from build123d import *

# Parameters (mm, degrees)
SKETCH1_R                        = 20
BOSS_EXTRUDE1_DEPTH              = 40
SKETCH1_3_R                      = 20
BOSS_EXTRUDE2_DEPTH              = 30
SKETCH2_W                        = 80
SKETCH2_H                        = 40
BOSS_EXTRUDE3_DEPTH              = 10
SKETCH6_W                        = 80
SKETCH6_H                        = 10
BOSS_EXTRUDE4_DEPTH              = 30
F_20_0MM_DOWEL_HOLE1_D           = 20
F_20_0MM_DOWEL_HOLE1_CSINK_D     = 20.05
F_20_0MM_DOWEL_HOLE1_CSINK_ANGLE = 90
SKETCH11_W                       = 60
SKETCH11_H                       = 100
BOSS_EXTRUDE5_DEPTH              = 10
FILLET1_R                        = 10
FILLET2_R                        = 10
CUT_EXTRUDE2_REACH               = 139.477


with BuildPart() as part:
    # Sketch1 → Boss-Extrude1 (new body)
    with BuildSketch(Plane.XY):
        with Locations((-40, 0)):
            Circle(SKETCH1_R)
    extrude(amount=BOSS_EXTRUDE1_DEPTH)



with BuildPart() as body_2:
    # Sketch1<3> → Boss-Extrude2 (new body)
    with BuildSketch(Plane.XY):
        with Locations((40, 0)):
            Circle(SKETCH1_3_R)
    extrude(amount=BOSS_EXTRUDE2_DEPTH)


with BuildPart() as part_1:
    add(part.part)

    add(body_2.part)  # Boss-Extrude3 merges body 2
    # Sketch2 → Boss-Extrude3 (add)
    with BuildSketch(Plane(origin=(0, 0, 0), x_dir=(-1, 0, 0), z_dir=(0, 0, -1))):
        Rectangle(SKETCH2_W, SKETCH2_H)
    extrude(amount=-BOSS_EXTRUDE3_DEPTH)

    # Sketch6 → Boss-Extrude4 (add)
    with BuildSketch(Plane.XY.offset(30)):
        with Locations((0, -15)):
            Rectangle(SKETCH6_W, SKETCH6_H)
    extrude(amount=-BOSS_EXTRUDE4_DEPTH)

    # Ø20.0mm Dowel Hole1 (through all)
    with Locations(Plane.XY.offset(40)):
        with Locations((-40, 0), (40.331351324, -0.177410636)):
            CounterSinkHole(F_20_0MM_DOWEL_HOLE1_D / 2, F_20_0MM_DOWEL_HOLE1_CSINK_D / 2, counter_sink_angle=F_20_0MM_DOWEL_HOLE1_CSINK_ANGLE)

    # Sketch11 → Boss-Extrude5 (add)
    with BuildSketch(Plane(origin=(0, 0, 0), x_dir=(-1, 0, 0), z_dir=(0, 0, -1))):
        with Locations((0, -70)):
            Rectangle(SKETCH11_W, SKETCH11_H)
    extrude(amount=-BOSS_EXTRUDE5_DEPTH)

    # Fillet1
    fillet1_edges = [part_1.edges().sort_by_distance(p)[0] for p in [
        (-30, -120, 5),
    ]]
    fillet(fillet1_edges, radius=FILLET1_R)

    # Fillet2
    fillet2_edges = [part_1.edges().sort_by_distance(p)[0] for p in [
        (30, -120, 5),
    ]]
    fillet(fillet2_edges, radius=FILLET2_R)

    # Sketch12 → Cut-Extrude2 (cut, up to next)
    with BuildSketch(Plane.XY.offset(10), mode=Mode.PRIVATE) as cut_extrude2_sk1:
        with BuildLine():
            Line((-5, -80), (10, -80))
            ThreePointArc((10, -80), (20, -90), (10, -100))
            Line((10, -100), (-5, -100))
            ThreePointArc((-5, -100), (-15, -90), (-5, -80))
        make_face()
    cut_extrude2_tool1 = extrude(cut_extrude2_sk1.sketch, amount=-CUT_EXTRUDE2_REACH, mode=Mode.PRIVATE) & part_1.part
    add(cut_extrude2_tool1.solids().sort_by_distance((2.5, -90, 10))[0], mode=Mode.SUBTRACT)


solid = part_1.part
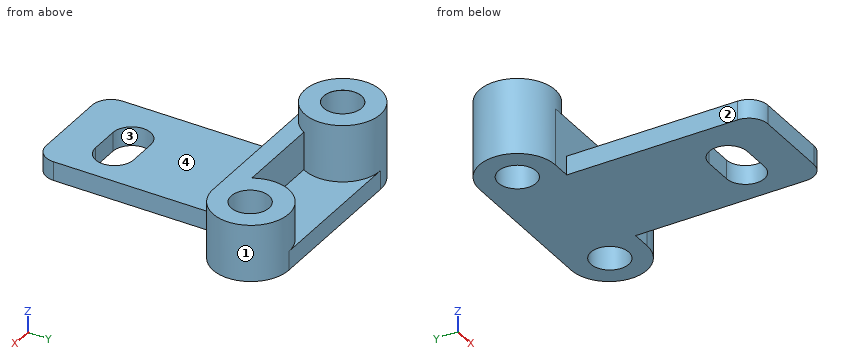
Read the model definition and answer for the solid it produces. Units are mm, in the model's axes. Face numbers are marked on the shaded views. A direction names the side the tool comes from. Round coordinates to 2 decimals unless told otherwise and drop trailing zeros. Order: outer loops, then holes, each group sorted by start corner. A loop starts at its lowest first (then second) coordinate and runs counter-clockwise, first axis right, second up.
1) The part is cut by section D-D on y = -24. Write down the section's boundary in (x, z).
2) The part is cut by section B-B on x = 43. Write down the section's boundary in (y, z), plus the area to 3 significant figures.
3) The part is cut by section C-C on z = 3. Write down the section's boundary in (x, y).
4) Flat-ended cylindrical pins translate along their axes: pin 1 (8 mm diameter, centred on x = 8.5, z = 25.5, fed in from -Y); pin 2 (20 mm diameter, centred on x = 5.5, y = 8.5, fed in from +Z); pin 3 (23 mm diameter, centred on x = 40.33, y = -0.18, fed in from +Z). Find the tip coordinate at first contact, or state that the pin passes through.
5) Straight lines are drawn through the part: L1, parallel to Y at x = -40, z = 24.5; L2, parallel to Z at x = 9, y = -69; L3, parallel to Y at x = -3, z = 15. For each, find the intervals that lie inside material, in ascending order.
6) The part is cut by section A-A on z = 37. Write down the section's boundary in (x, y).
7) For the marked faces 1, 2, 3 and 4, determine the directions among +Z, -Z, +X, -X, +Y, -Y from which every point of the face is accessible in a straight line to the end or side of a thin tool.
Resolved:
1. outline: (-30, 0) - (30, 0) - (30, 10) - (-30, 10) - close
2. outline: (-19.77, 0) - (-9.81, 0) - (-9.81, 30) - (-19.77, 30) - close; (9.46, 0) - (19.77, 0) - (19.77, 30) - (9.46, 30) - close
2. area: 608 mm2
3. outline: (-40, -20) - (-30, -20) - (-30, -110) arc R10 ccw to (-20, -120) - (20, -120) arc R10 ccw to (30, -110) - (30, -20) - (40, -20) arc R20 ccw to (40, 20) - (-40, 20) arc R20 ccw to start; hole circle Ø20 at (-40, 0); hole (-5, -100) - (10, -100) arc R10 ccw to (10, -80) - (-5, -80) arc R10 ccw to start; hole circle Ø20 at (40.33, -0.18)
4. pin 1: stops at y = -20
4. pin 2: stops at z = 10
4. pin 3: stops at z = 30
5. L1: y = -20 to -10, 10 to 20
5. L2: z = 0 to 10
5. L3: y = -20 to -10
6. outline: circle Ø40 at (-40, 0); hole circle Ø20 at (-40, 0)
7. face 1: +Z
7. face 2: +Z, -Z, -X, -Y
7. face 3: +Z, -Z
7. face 4: +Z, +X, -X, -Y
